The listing builds one solid part. Answer for the finished solid, in the listing's coordinates (mm). A direction names the side the tool comes from. Round coordinates to 2 decimals unless told otherwise and drop trailing zeros. Order: outer loops, then holes, each group sorted by start corner. A loop starts at its lowest first (then second) coordinate and runs counter-clockwise, first axis right, second up. Notation, with made-up numbers: (39, 68) -> (81, 68) arc R23 cw to (81, 86) -> close; hole circle Ø7 at (-11.75, -16). An arc over 180 degrees is marked (long way). Return JSON: item names as keys, results as strings. Group by question number.
(1) The part is cut by section A-A (z = 0). Determine the outline of the cut face in (x, y).
(2) The part is cut by section D-D (x = 5). Determine the outline of the cut face in (y, z), plus the area to 3 significant figures.
(3) Determine the mould class of faces 1 (the face through (-11, -2, 1)), 2 (the face through (-2, -1, 16)), 3 (the face through (10, 2, -1)) for opening direction X: +X half, -X half, draft (parallel to the pull), parting line (faces both ways), or undercut.
(4) The part is cut by section C-C (z = -44.45). Determine the outline of the cut face in (x, y).
(5) Each of these flat-tipped pins is pushed along its axis until it touches: pin 1 (3.5 mm diameter, centred on x = -13.57, z = -6.4, fed in from +Y); pin 2 (1.5 mm diameter, centred on x = 18.5, y = 1, fed in from -Z); pin 3 (2 mm diameter, centred on y = 3, z = -19.5, fed in from +X). Where does it stop, or does it pass through?
(6) The part is cut by section B-B (x = -20.5). Determine the outline of the cut face in (y, z).
(7) Which of the six approach directions +Z, -Z, +X, -X, +Y, -Y give full straight-line access (tool end or side, diameter ignored) to faces 4 (the face through (0, 4, 44)), 5 (the face through (-52.53, 3.43, 4.85)), 6 (the face through (-0.55, -1.49, 13.49))?
(8) Consider line 1 (Z direction, x = 0, y = -0.5); line 2 (X direction, y = 1.4, z = 0); line 3 (Z direction, x = -2.5, y = 1.5). Determine where each line is inside the solid, lowest interval first. Write a range as [from, to].
from build123d import *

# Parameters (mm, degrees)
SKETCH1_R           = 53.5
BOSS_EXTRUDE1_DEPTH = 2
SKETCH2_R           = 2.7
BOSS_EXTRUDE2_DEPTH = 2
SKETCH3_R           = 3.55
CUT_EXTRUDE1_DEPTH  = 2
SKETCH7_R           = 53.5
SKETCH7_R_2         = 52
BOSS_EXTRUDE3_DEPTH = 10
SKETCH8_W           = 56.651812746
SKETCH8_H           = 12.7
CUT_EXTRUDE4_DEPTH  = 10
SKETCH13_R          = 53.5
SKETCH13_R_2        = 3.55
BOSS_EXTRUDE4_DEPTH = 2
SKETCH12_R          = 2.8
CUT_EXTRUDE6_DEPTH  = 3
SKETCH16_R          = 1.5
CUT_EXTRUDE8_DEPTH  = 77.769134423
FILLET3_R           = 5


with BuildPart() as part:
    # Sketch1 → Boss-Extrude1 (new body)
    with BuildSketch(Plane(origin=(0, 0, 0), x_dir=(1, 0, 0), z_dir=(0, 1, 0))):
        with Locations(Location((0, 0, 0), (0, 0, 270))):
            Circle(SKETCH1_R)
    extrude(amount=BOSS_EXTRUDE1_DEPTH)

    # Sketch2 → Boss-Extrude2 (add)
    with BuildSketch(Plane(origin=(0, 2, 0), x_dir=(1, 0, 0), z_dir=(0, 1, 0))):
        with Locations(Location((0, -44.45, 0), (0, 0, 270))):
            Circle(SKETCH2_R)
        with Locations(Location((0, 44.45, 0), (0, 0, 270))):
            Circle(SKETCH2_R)
    extrude(amount=BOSS_EXTRUDE2_DEPTH)

    # Sketch3 → Cut-Extrude1 (cut)
    with BuildSketch(Plane(origin=(0, 2, 0), x_dir=(1, 0, 0), z_dir=(0, 1, 0))):
        with Locations(Location((0, 0, 0), (0, 0, 270))):
            Circle(SKETCH3_R)
    extrude(amount=-CUT_EXTRUDE1_DEPTH, mode=Mode.SUBTRACT)

    # Sketch7 → Boss-Extrude3 (add)
    with BuildSketch(Plane(origin=(0, 2, 0), x_dir=(1, 0, 0), z_dir=(0, 1, 0))):
        with Locations(Location((0, 0, 0), (0, 0, 270))):
            Circle(SKETCH7_R)
        with Locations(Location((0, 0, 0), (0, 0, 270))):
            Circle(SKETCH7_R_2, mode=Mode.SUBTRACT)
    extrude(amount=BOSS_EXTRUDE3_DEPTH)

    # Sketch8 → Cut-Extrude4 (cut)
    with BuildSketch(Plane(origin=(0, 2, 0), x_dir=(1, 0, 0), z_dir=(0, 1, 0))):
        with Locations((-28.325906373, 0)):
            Rectangle(SKETCH8_W, SKETCH8_H)
    extrude(amount=CUT_EXTRUDE4_DEPTH, mode=Mode.SUBTRACT)

    # Sketch13 → Boss-Extrude4 (add)
    with BuildSketch(Plane.XZ):
        with Locations(Location((0, 0, 0), (0, 0, 270))):
            Circle(SKETCH13_R)
        with Locations(Location((0, 0, 0), (0, 0, 90))):
            Circle(SKETCH13_R_2, mode=Mode.SUBTRACT)
    extrude(amount=BOSS_EXTRUDE4_DEPTH)

    # Sketch12 → Cut-Extrude6 (cut)
    with BuildSketch(Plane(origin=(0, 2, 0), x_dir=(1, 0, 0), z_dir=(0, 1, 0))):
        with Locations(Location((11.16900504, 10.012658309, 0), (0, 0, 270))):
            Circle(SKETCH12_R)
        with Locations(Location((-0.61610798, -14.987341691, 0), (0, 0, 270))):
            Circle(SKETCH12_R)
        with Locations(Location((-13.568010506, 6.396021491, 0), (0, 0, 270))):
            Circle(SKETCH12_R)
    extrude(amount=-CUT_EXTRUDE6_DEPTH, mode=Mode.SUBTRACT)

    # Sketch16 → Cut-Extrude8 (cut, through all)
    with BuildSketch(Plane(origin=(0, -1, 0), x_dir=(1, 0, 0), z_dir=(0, 1, 0))):
        with Locations(Location((11.16900504, 10.012658309, 0), (0, 0, 270))):
            Circle(SKETCH16_R)
        with Locations(Location((-0.61610798, -14.987341691, 0), (0, 0, 270))):
            Circle(SKETCH16_R)
        with Locations(Location((-13.568010506, 6.396021491, 0), (0, 0, 270))):
            Circle(SKETCH16_R)
    extrude(amount=-CUT_EXTRUDE8_DEPTH, mode=Mode.SUBTRACT)

    # Fillet3
    fillet3_edges = [part.edges().sort_by_distance(p)[0] for p in [
        (-52.366322452, 12, -6.35),
        (-52.366322452, 12, 6.35),
        (-52.366322452, 2, 6.35),
        (-52.366322452, 2, -6.35),
    ]]
    fillet(fillet3_edges, radius=FILLET3_R - 0.0001)  # a hair under: the kernel refuses the full size


solid = part.part
Answer below:
{
 "1": {"outline": "(-53.5, -2) -> (-3.55, -2) -> (-3.55, 2) -> (-53.5, 2) -> close; (3.55, -2) -> (53.5, -2) -> (53.5, 12) -> (52, 12) -> (52, 2) -> (3.55, 2) -> close"},
 "2": {"outline": "(-2, -53.27) -> (12, -53.27) -> (12, -51.76) -> (2, -51.76) -> (2, 51.76) -> (12, 51.76) -> (12, 53.27) -> (-2, 53.27) -> close", "area": "456 mm²"},
 "3": {"face 1": "draft", "face 2": "undercut", "face 3": "undercut"},
 "4": {"outline": "(-29.77, -2) -> (29.77, -2) -> (29.77, 12) -> (26.99, 12) -> (26.99, 2) -> (2.7, 2) -> (2.7, 4) -> (-2.7, 4) -> (-2.7, 2) -> (-26.99, 2) -> (-26.99, 12) -> (-29.77, 12) -> close"},
 "5": {"pin 1": "stops at y = -1", "pin 2": "stops at z = -50.47", "pin 3": "stops at x = 50.2"},
 "6": {"outline": "(-2, -49.42) -> (12, -49.42) -> (12, -47.79) -> (2, -47.79) -> (2, 47.79) -> (12, 47.79) -> (12, 49.42) -> (-2, 49.42) -> close"},
 "7": {"face 4": "+Y", "face 5": "-X, +Y", "face 6": "+Y, -Y"},
 "8": {"line 1": "z = [-53.5, -3.55], [3.55, 12.26], [17.72, 53.5]", "line 2": "x = [-53.5, -3.55], [3.55, 53.5]", "line 3": "z = [-53.44, -2.52], [2.52, 12.92], [17.06, 53.44]"}
}
